The figure shows three views and two pictorial views of one solid part (mm, origin at its lowest corner). Answer the questions. Give positions to 0.01 mm unless a question says otherwise; leave off trailing zeros. Write each loop counter-clockwise with the first axis right and the second up, starting at its lowest first coordinate (ties: lowest second). Pieces come first, ordered by that corner, then holes. Notation, with made-up numbers: (-8.5, -31.75) - (15.5, -31.75) arc R18 ccw to (15.5, -13.75) - close; hole circle Ø11 at (59.5, -32.5). An arc over 180 degrees is marked (long way). One line per question, with ' | ' between items. Start each with the question number.
1. The mould has two halves that part along Y. Classify the marked faces 1, 2 and 3: +Y half, -Y half, draft (parallel to the pull), parting line (faces both ways), or undercut.
2. Given P1, Ø1, axis at y = 11, z = 4, coming from the +X side; P2, Ø2, axis at y = 11, z = 4, coming from the +X side; P3, Ø2.5, axis at x = 7.5, y = 7.5, coming from the -Z side; P4, Ø4, axis at x = 11, z = 4.5, coming from the +Y side, each flat-ended and moving along its own axis, determine where each tip first touches the part or whether it passes through.
3. Find the intervals of material crossed by L1, parallel to Y at x = 7.5, z = 7; L2, parallel to Y at x = 4.5, z = 4; L3, parallel to X at y = 3.75, z = 4.25, in increasing order. Write a range as from..to.
4. A cutting plane is placed at C-C (z = 6.5). Determine the outline of the cut face in (x, y), then the cut area to 3 significant figures.
5. A cutting plane is placed at A-A (y = 7.5). Determine the outline of the cut face in (x, z).
6. A cutting plane is placed at D-D (z = 9). Determine the outline of the cut face in (x, y).
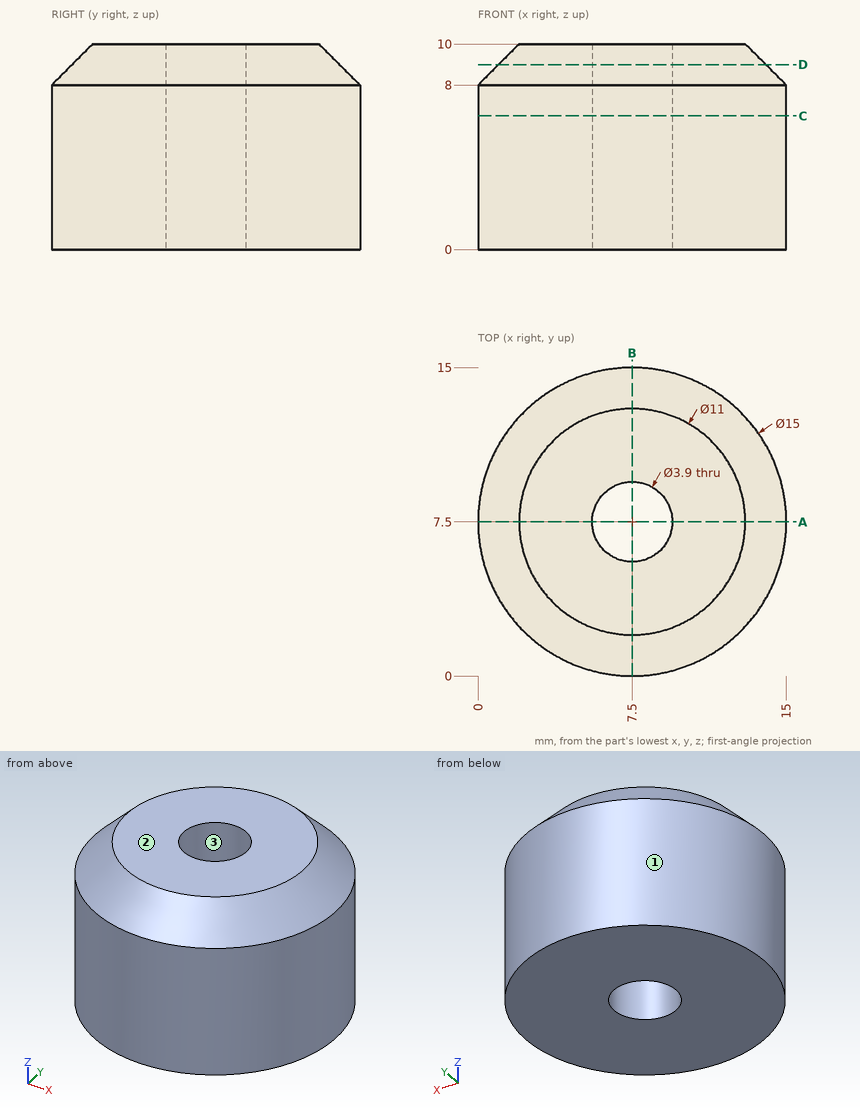
Determined:
1) face 1: parting line | face 2: draft | face 3: undercut
2) P1: x = 14.37 | P2: x = 14.57 | P3: through | P4: y = 14.85
3) L1: 0..5.55, 9.45..15 | L2: 0.63..14.37 | L3: 1..14
4) outline: circle Ø15 at (7.5, 7.5); hole circle Ø3.9 at (7.5, 7.5) | area: 165 mm2
5) outline: (0, 0) - (5.55, 0) - (5.55, 10) - (2, 10) - (0, 8) - close; (9.45, 0) - (15, 0) - (15, 8) - (13, 10) - (9.45, 10) - close
6) outline: circle Ø13 at (7.5, 7.5); hole circle Ø3.9 at (7.5, 7.5)
